```python
from build123d import *

# Parameters (mm, degrees)
SKETCH1_R           = 7.5
BOSS_EXTRUDE1_DEPTH = 15
BOSS_EXTRUDE2_DEPTH = 9.5
CUT_EXTRUDE1_DEPTH  = 12


with BuildPart() as part:
    # Sketch1 → Boss-Extrude1 (new body)
    with BuildSketch(Plane(origin=(0, 0, 0), x_dir=(1, 0, 0), z_dir=(0, 1, 0))):
        Circle(SKETCH1_R)
    extrude(amount=BOSS_EXTRUDE1_DEPTH)

    # Sketch4 → Boss-Extrude2 (add)
    with BuildSketch(Plane(origin=(0, 15, 0), x_dir=(1, 0, 0), z_dir=(0, 1, 0))):
        Polygon((1.934123402, 3.35), (-1.934123402, 3.35), (-3.868246804, 0), (-1.934123402, -3.35), (1.934123402, -3.35), (3.868246804, 0), align=None)
    extrude(amount=BOSS_EXTRUDE2_DEPTH)

    # Sketch5 → Cut-Extrude1 (cut)
    with BuildSketch(Plane.XZ):
        with BuildLine():
            Line((1.696172161, 2.627), (-1.696172161, 2.627))
            ThreePointArc((-1.696172161, 2.627), (-1.495693594, -2.74609353), (3.127, 0))
            ThreePointArc((3.127, 0), (2.74609353, 1.495693594), (1.696172161, 2.627))
        make_face()
    extrude(amount=-CUT_EXTRUDE1_DEPTH, mode=Mode.SUBTRACT)


solid = part.part
```
CAD build for the part. Positions are in the model's coordinates, mm. A direction names the side the tool comes from. Give positions to 0.01 mm unless a question says otherwise; leave off trailing zeros. Write each loop counter-clockwise with the first axis right and the second up, starting at its lowest first coordinate (ties: lowest second). Pieces come first, ordered by that corner, then holes. Notation, with made-up numbers: (-29.75, 7.5) -> (19.25, 7.5) arc R16 cw to (19.25, 14.5) -> close; hole circle Ø3 at (21.25, 36). An arc over 180 degrees is marked (long way). Write each question's results on one line, items separated by ' | '.
1. Cut at A-A, the plane x = 0. Write the cut outline in (y, z).
Geometry check:
outline: (0, -7.5) -> (15, -7.5) -> (15, -3.35) -> (24.5, -3.35) -> (24.5, 3.35) -> (15, 3.35) -> (15, 7.5) -> (0, 7.5) -> (0, 2.63) -> (12, 2.63) -> (12, -3.13) -> (0, -3.13) -> close
2. Cut at B-B, the plane z = -2.25. Write the cut outline in (x, y).
Geometry check:
outline: (-7.15, 0) -> (-2.17, 0) -> (-2.17, 12) -> (2.17, 12) -> (2.17, 0) -> (7.15, 0) -> (7.15, 15) -> (2.57, 15) -> (2.57, 24.5) -> (-2.57, 24.5) -> (-2.57, 15) -> (-7.15, 15) -> close
3. Drop flat-ended pins along their axis: P1, Ø4, axis at x = 4.5, y = 16, coming from the +Z side; P2, Ø6, axis at y = 5, z = 4, coming from the -X side; P3, Ø1.2, axis at x = -0.5, y = 18, coming from the +Z side. Give the stop position or say it passes through.
Geometry check:
P1: z = 6.97 | P2: x = -7.43 | P3: z = 3.35
4. Cut at D-D, the plane z = -4.5. Write the cut outline in (x, y).
Geometry check:
outline: (-6, 0) -> (6, 0) -> (6, 15) -> (-6, 15) -> close
5. Two-plate mould, pull along Z, no slides. Class faces 4 (the flat face through (0, 12, 0)), 5 (the flat face through (3, 15, 2)), 6 (the flat face through (-2.888, 19.684, -1.698)): pulls with the +Z half, pulls with the -Z half, needs draft (parallel to the pull), parting line crosses it, or undercut.
Geometry check:
face 4: undercut | face 5: needs draft | face 6: pulls with the -Z half
6. Cut at C-C, the plane y = 18. Write the cut outline in (x, z).
Geometry check:
outline: (-3.87, 0) -> (-1.93, -3.35) -> (1.93, -3.35) -> (3.87, 0) -> (1.93, 3.35) -> (-1.93, 3.35) -> close
7. Wall check: probe 1 along Z at (x, y) = (0, 9.5); probe 2 along X at (y, z) = (4, 0); probe 3 along Z at (x, y) = (0.5, 19.75). Give the ranges that are in metal, low to high. Write a range as [from, to].
Geometry check:
probe 1: [-7.5, -3.13], [2.63, 7.5] | probe 2: [-7.5, -3.13], [3.13, 7.5] | probe 3: [-3.35, 3.35]
8. Which spindle directions (+Z, -Z, +X, -X, +Y, -Y) get a long thin tool onto all of the face, cutting with end or side? Do faces 1 (the flat face through (0, 6, 2.627)), 2 (the flat face through (0, 20, -3.35)), 3 (the flat face through (2.915, 19.684, -1.652)). Say none if no direction does.
Geometry check:
face 1: -Y | face 2: -Z, +X, -X, +Y | face 3: -Z, +X, +Y
